Source: CAD feature listing. Evaluate the final solid. Frame: model axes, mm. A direction names the side the tool comes from. Coordinates: 2 decimals unless noted, no trailing zeros. Loops run counter-clockwise (first coordinate to the right, second up) from the corner with the lowest first, then second, coordinate; pieces in that order, holes last.
```python
from build123d import *

# Parameters (mm, degrees)
F1_DEPTH    = 8
F4_DEPTH    = 12
F5_DEPTH    = 12
F6_DEPTH    = 4
F7_T2_ANGLE = 226.9097490639
F7_T4_ANGLE = 226.9097490639
F8_R        = 2


# Not quite as in the source:
# - a fillet or chamfer that OpenCascade refuses, or shapes differently, is made with other operations: its cross-section is extruded or revolved along the edge and cut away or added
# - a feature names something its author has since deleted; it is built from what else it names


with BuildPart() as f1:
    # F0 (on Top) → F1 (new body)
    with BuildSketch(Plane.XY):
        with BuildLine():
            ThreePointArc((-26.2934756426, -6.4967182246), (-21.8313594954, -4.5225872947), (-20, 0))
            ThreePointArc((-20, 0), (-21.8313594954, 4.5225872947), (-26.2934756426, 6.4967182246))
            ThreePointArc((-26.2934756426, 6.4967182246), (-33, 0), (-26.2934756426, -6.4967182246))
        make_face()
        with BuildLine():
            ThreePointArc((4.9180788932, 0), (0, 2.25), (-4.9180788932, 0))
            ThreePointArc((-4.9180788932, 0), (0, -2.25), (4.9180788932, 0))
        make_face()
        with BuildLine():
            Line((6.4380174247, 0), (6.3926786471, 3.0737093407))
            ThreePointArc((6.3926786471, 3.0737093407), (5.8604804677, 1.4384579519), (4.9180788932, 0))
            ThreePointArc((4.9180788932, 0), (6.0748085227, -1.9377064606), (6.4992929884, -4.1541321195))
            Line((6.4992929884, -4.1541321195), (6.4380174247, 0))
        make_face()
        with BuildLine():
            ThreePointArc((-26.2934756426, 6.4967182246), (-21.8313594954, 4.5225872947), (-20, 0))
            ThreePointArc((-20, 0), (-21.8313594954, -4.5225872947), (-26.2934756426, -6.4967182246))
            Line((-26.2934756426, -6.4967182246), (-6.0993653128, -6.4967182246))
            ThreePointArc((-6.0993653128, -6.4967182246), (-6.3951431673, -3.0871827877), (-4.9180788932, 0))
            ThreePointArc((-4.9180788932, 0), (-6.3951431673, 3.0871827877), (-6.0993653128, 6.4967182246))
            Line((-6.0993653128, 6.4967182246), (-26.2934756426, 6.4967182246))
        make_face()
        with BuildLine():
            ThreePointArc((-4.9180788932, 0), (-6.3951431673, -3.0871827877), (-6.0993653128, -6.4967182246))
            ThreePointArc((-6.0993653128, -6.4967182246), (1.141079635, -10.6490575296), (6.5, -4.25))
            ThreePointArc((6.5, -4.25), (6.4998232447, -4.2020647563), (6.4992929884, -4.1541321195))
            ThreePointArc((6.4992929884, -4.1541321195), (6.0748085227, -1.9377064606), (4.9180788932, 0))
            ThreePointArc((4.9180788932, 0), (0, -2.25), (-4.9180788932, 0))
        make_face()
        with BuildLine():
            ThreePointArc((6.3552032224, 5.614328407), (0.4593650036, 10.7337476658), (-6.0993653128, 6.4967182246))
            ThreePointArc((-6.0993653128, 6.4967182246), (-6.3951431673, 3.0871827877), (-4.9180788932, 0))
            ThreePointArc((-4.9180788932, 0), (0, 2.25), (4.9180788932, 0))
            ThreePointArc((4.9180788932, 0), (5.8604804677, 1.4384579519), (6.3926786471, 3.0737093407))
            Line((6.3926786471, 3.0737093407), (6.3552032224, 5.614328407))
        make_face()
        with BuildLine():
            ThreePointArc((6.5, 4.25), (6.4636994417, 4.9359952822), (6.3552032224, 5.614328407))
            Line((6.3552032224, 5.614328407), (6.3926786471, 3.0737093407))
            ThreePointArc((6.3926786471, 3.0737093407), (6.4731140576, 3.6594118212), (6.5, 4.25))
        make_face()
    extrude(amount=F1_DEPTH)



with BuildPart() as f4:
    # F3 (on line) → F4 (new body)
    with BuildSketch(Plane(origin=(0.4312653925, -1.6095043562, 0), x_dir=(-0.9659258263, -0.2588190451, 0), z_dir=(-0.2588190451, 0.9659258263, 0))):
        with BuildLine():
            Line((-79.4407832557, 0), (-74.9686473007, 0))
            Line((-74.9686473007, 0), (-74.9686473007, 8))
            Line((-74.9686473007, 8), (-79.4407832557, 8))
            ThreePointArc((-79.4407832557, 8), (-80.9686473007, 4), (-79.4407832557, 0))
        make_face()
        with BuildLine():
            Line((-74.9686473007, 8), (-74.9686473007, 0))
            Line((-74.9686473007, 0), (-70.4965113457, 0))
            ThreePointArc((-70.4965113457, 0), (-69.3636131469, 1.8590674614), (-68.9686473007, 4))
            ThreePointArc((-68.9686473007, 4), (-69.3636131469, 6.1409325386), (-70.4965113457, 8))
            Line((-70.4965113457, 8), (-74.9686473007, 8))
        make_face()
    extrude(amount=F4_DEPTH)


with BuildPart() as f5:
    # F3 (on line) → F5 (new body)
    with BuildSketch(Plane(origin=(0.4312653925, -1.6095043562, 0), x_dir=(-0.9659258263, -0.2588190451, 0), z_dir=(-0.2588190451, 0.9659258263, 0))):
        with BuildLine():
            ThreePointArc((-54.2186473007, 6.5), (-56.7186473007, 4), (-54.2186473007, 1.5))
            Line((-54.2186473007, 1.5), (-54.2186473007, 4))
            Line((-54.2186473007, 4), (-54.2186473007, 6.5))
        make_face()
        with BuildLine():
            ThreePointArc((-51.7186473007, 4), (-52.4508803477, 5.767766953), (-54.2186473007, 6.5))
            Line((-54.2186473007, 6.5), (-54.2186473007, 4))
            Line((-54.2186473007, 4), (-51.7186473007, 4))
        make_face()
        with BuildLine():
            Line((-54.2186473007, 4), (-54.2186473007, 1.5))
            ThreePointArc((-54.2186473007, 1.5), (-52.4508803477, 2.232233047), (-51.7186473007, 4))
            Line((-51.7186473007, 4), (-54.2186473007, 4))
        make_face()
    extrude(amount=F5_DEPTH)


with BuildPart() as f1_1:
    add(f1.part)

    add(f4.part)  # F6 merges F4

    add(f5.part)  # F6 merges F5
    # F3 (on line) → F6 (join)
    with BuildSketch(Plane(origin=(0.4312653925, -1.6095043562, 0), x_dir=(-0.9659258263, -0.2588190451, 0), z_dir=(-0.2588190451, 0.9659258263, 0))):
        with BuildLine():
            Line((-54.2186473007, 1.5), (-54.2186473007, 0))
            Line((-54.2186473007, 0), (-6.2186473007, 0))
            Line((-6.2186473007, 0), (-6.2186473007, 4))
            Line((-6.2186473007, 4), (-51.7186473007, 4))
            ThreePointArc((-51.7186473007, 4), (-52.4508803477, 2.232233047), (-54.2186473007, 1.5))
        make_face()
        with BuildLine():
            Line((-6.2186473007, 8), (-54.2186473007, 8))
            Line((-54.2186473007, 8), (-54.2186473007, 6.5))
            ThreePointArc((-54.2186473007, 6.5), (-52.4508803477, 5.767766953), (-51.7186473007, 4))
            Line((-51.7186473007, 4), (-6.2186473007, 4))
            Line((-6.2186473007, 4), (-6.2186473007, 8))
        make_face()
        with BuildLine():
            ThreePointArc((-68.9686473007, 4), (-69.3636131469, 1.8590674614), (-70.4965113457, 0))
            Line((-70.4965113457, 0), (-54.2186473007, 0))
            Line((-54.2186473007, 0), (-54.2186473007, 1.5))
            ThreePointArc((-54.2186473007, 1.5), (-56.7186473007, 4), (-54.2186473007, 6.5))
            Line((-54.2186473007, 6.5), (-54.2186473007, 8))
            Line((-54.2186473007, 8), (-70.4965113457, 8))
            ThreePointArc((-70.4965113457, 8), (-69.3636131469, 6.1409325386), (-68.9686473007, 4))
        make_face()
    extrude(amount=F6_DEPTH)

    # F7: fillet of radius 3 on 2 edges, made by hand

    # F7_s1 → F7_t2 (revolve, cut)
    with BuildSketch(Plane(origin=(62.3527130216, 16.7073591, 28.0076976241), x_dir=(-0.2588190451, 0.9659258263, 0), z_dir=(0.8861150843, 0.2374338212, 0.3980266798))):
        with BuildLine():
            ThreePointArc((7.3337184778, -32.1700264164), (9.4550388213, -31.2913467599), (10.3337184778, -29.1700264164))
            Line((10.3337184778, -29.1700264164), (10.3337184778, -32.1700264164))
            Line((10.3337184778, -32.1700264164), (7.3337184778, -32.1700264164))
        make_face()
    revolve(axis=Axis((69.7395894409, 29.3849192663, 4), (-0.2588190451, 0.9659258263, 0)), revolution_arc=F7_T2_ANGLE, mode=Mode.SUBTRACT)

    # F7_s3 → F7_t4 (revolve, cut)
    with BuildSketch(Plane(origin=(62.3527130216, 16.7073591, 28.0076976241), x_dir=(0.2588190451, -0.9659258263, 0), z_dir=(-0.8861150843, -0.2374338212, -0.3980266798))):
        with BuildLine():
            ThreePointArc((-7.3337184778, -20.1700264164), (-9.4550388213, -21.0487060728), (-10.3337184778, -23.1700264164))
            Line((-10.3337184778, -23.1700264164), (-10.3337184778, -20.1700264164))
            Line((-10.3337184778, -20.1700264164), (-7.3337184778, -20.1700264164))
        make_face()
    revolve(axis=Axis((69.7395894409, 29.3849192663, 4), (-0.2588190451, 0.9659258263, 0)), revolution_arc=F7_T4_ANGLE, mode=Mode.SUBTRACT)

    # F8
    f8_edges = [f1_1.edges().sort_by_distance(p)[0] for p in [
        (49.696629, 24.014424, 6.5),
    ]]
    fillet(f8_edges, radius=F8_R)

    # F9: F1 across plane


with BuildPart() as f1_2:
    add(f1_1.part)
    add(f1_1.part.mirror(Plane.XZ))


solid = f1_2.part
```
Q1. Reachability of faces 4 (the flat face through (-16, -6.497, 4)), 5 (the flat face through (-16, 6.497, 4)), 6 (the flat face through (18, 4, 0)), 7 (the flat face through (43.045, 9.809, 4.056)) from +Z, -Z, +X, -X, +Y, -Y: full face, straight path, thin tool, end or side. Return the list, or none.
Q2. Section query D-D on x = 2. Return the cut outline in (y, z).
Q3. Section query A-A on y = -8. Return the cut outline in (x, z), then the cut area to 3 significant figures.
Q4. Material intervals for line 1 along Y through (x, z) = (-18, 2.5); line 2 along Y through (x, z) = (16.5, 3.75); line 3 along Y through (x, z) = (21.5, 1.5), sorted ascending.
Q5. First-contact query: pin 1 Ø1 at (x, z) = (63, 4) entering from +Y; pin 2 Ø2.5 at (x, z) = (-18, 2.5) entering from +Y; pin 3 Ø4 at (x, z) = (-19, 3) entering from -Y. Flat tips, straight axial feed; report the tip coordinate or a pass-through.
Q6. Section query C-C on x = -21. Return the cut outline in (y, z).
Q7. Draft query along Y for faces 1 (the flat face through (43.045, -9.809, 4.056)), 2 (the cylindrical face through (-33, 0, 4)), 3 (the cylindrical face through (77.5, -23.6, 4.1)). Return one class per face: released by +Y, released by -Y, zero draft, split by the parting line, or undercut.
Q8. Section query B-B on x = 41.5. Return the cut outline in (y, z).
Resolved:
1. face 4: +Z, -Z, -X, -Y
1. face 5: +Z, -Z, -X, +Y
1. face 6: -Z, +X, -X, +Y, -Y
1. face 7: +Z, -Z, +X
2. outline: (-10.43, 0) - (10.43, 0) - (10.43, 8) - (-10.43, 8) - close
3. outline: (-5.31, 0) - (5.31, 0) - (5.31, 8) - (-5.31, 8) - close; (20.84, 0) - (36.29, 0) - (36.29, 8) - (20.84, 8) - close
3. area: 209 mm2
4. line 1: y = -6.5 to 6.5
4. line 2: y = -6.84 to -2.7, 2.7 to 6.84
4. line 3: y = -8.18 to -4.04, 4.04 to 8.18
5. pin 1: stops at y = 19.43
5. pin 2: stops at y = 6.5
5. pin 3: stops at y = -6.5
6. outline: (-6.5, 0) - (6.5, 0) - (6.5, 8) - (-6.5, 8) - close
7. face 1: undercut
7. face 2: split by the parting line
7. face 3: released by -Y
8. outline: (-13.54, 0) - (-9.39, 0) - (-9.39, 8) - (-13.54, 8) - close; (9.39, 0) - (13.54, 0) - (13.54, 8) - (9.39, 8) - close
